Verification items for the finished model (mm, model axes). Face numbers are marked on the shaded views. A direction names the side the tool comes from. Coordinates: 2 decimals unless noted, no trailing zeros. Loops run counter-clockwise (first coordinate to the right, second up) from the corner with the lowest first, then second, coordinate; pieces in that order, holes last.
Q1. Sectioned sample at B-B (x = 10). Enter the section's corners in (y, z).
Q2. Mould release check, pull along X, two halves, no side actions. Record for the marked faces 1, 2 and 3: +X half, -X half, draft (parallel to the pull), parting line (faces both ways), or undercut.
Q3. Sectioned sample at A-A (y = 7.25). Enter the section's corners in (x, z), then the cut area to 3 significant figures.
Q4. Sectioned sample at D-D (x = 20). Enter the section's corners in (y, z), then the cut area to 3 significant figures.
Q5. Material ranges on probe 1 along X at (y, z) = (1, 0); probe 2 along X at (y, z) = (11, 3.55); probe 3 along Z at (x, y) = (6.75, 11.25), recorded low to high.
Q6. Sectioned sample at C-C (y = 3.5). Enter the section's corners in (x, z), then the cut area to 3 significant figures.
Q7. Go/stop test with flat-tipped pins: P1, Ø4, axis at x = 10, y = 11, coming from the +Z side; P2, Ø7, axis at x = 10, y = 11, coming from the -Z side; P3, Ø5, axis at x = 10.5, y = 11, coming from the +Z side; P4, Ø1.5, axis at y = 8, z = 3.5, coming from the +X side. Record where each tip stops, or that it passes through.
Q8. Access from +Z, -Z, +X, -X, +Y, -Y to the whole of each face (thin tool, end or side, straight path). Record for the marked faces 4, 5, 6, 7 and 8.
```python
from build123d import *

# Parameters (mm, degrees)
SKETCH1_W           = 10
SKETCH1_H           = 10
SKETCH1_R           = 2.05
BOSS_EXTRUDE1_DEPTH = 6
CUT_EXTRUDE1_DEPTH  = 3.2
SKETCH3_W           = 10
SKETCH3_H           = 6
BOSS_EXTRUDE2_DEPTH = 20
SKETCH4_R           = 2.05
CUT_EXTRUDE2_DEPTH  = 27.191601707
CUT_EXTRUDE3_DEPTH  = 3.2
SKETCH8_R           = 2.2
BOSS_EXTRUDE4_DEPTH = 4.5
SKETCH10_W          = 17.254554438
SKETCH10_H          = 12.252832867
CUT_EXTRUDE5_DEPTH  = 1.6


with BuildPart() as part:
    # Sketch1 → Boss-Extrude1 (new body)
    with BuildSketch(Plane(origin=(0, 0, 0), x_dir=(1, 0, 0), z_dir=(0, 1, 0))):
        Rectangle(SKETCH1_W, SKETCH1_H)
        with Locations(Location((0, 0, 0), (0, 0, 270))):
            Circle(SKETCH1_R, mode=Mode.SUBTRACT)
    extrude(amount=BOSS_EXTRUDE1_DEPTH)

    # Sketch2 → Cut-Extrude1 (cut)
    with BuildSketch(Plane(origin=(0, 6, 0), x_dir=(1, 0, 0), z_dir=(0, 1, 0))):
        Polygon((4.041451884, 0), (2.020725942, 3.5), (-2.020725942, 3.5), (-4.041451884, 0), (-2.020725942, -3.5), (2.020725942, -3.5), align=None)
    extrude(amount=-CUT_EXTRUDE1_DEPTH, mode=Mode.SUBTRACT)

    # Sketch3 → Boss-Extrude2 (add)
    with BuildSketch(Plane(origin=(5, 0, 0), x_dir=(0, 0, -1), z_dir=(1, 0, 0))):
        with Locations((0, 3)):
            Rectangle(SKETCH3_W, SKETCH3_H)
    extrude(amount=BOSS_EXTRUDE2_DEPTH)

    # Sketch4 → Cut-Extrude2 (cut, through all)
    with BuildSketch(Plane(origin=(0, 6, 0), x_dir=(1, 0, 0), z_dir=(0, 1, 0))):
        with Locations(Location((20, 0, 0), (0, 0, 270))):
            Circle(SKETCH4_R)
    extrude(amount=-CUT_EXTRUDE2_DEPTH, mode=Mode.SUBTRACT)

    # Sketch5 → Cut-Extrude3 (cut)
    with BuildSketch(Plane(origin=(0, 6, 0), x_dir=(1, 0, 0), z_dir=(0, 1, 0))):
        Polygon((24.041451884, 0), (22.020725942, 3.5), (17.979274058, 3.5), (15.958548116, 0), (17.979274058, -3.5), (22.020725942, -3.5), align=None)
    extrude(amount=-CUT_EXTRUDE3_DEPTH, mode=Mode.SUBTRACT)

    # Sketch8 → Boss-Extrude4 (add, symmetric)
    with BuildSketch(Plane.XY):
        with BuildLine():
            Line((5, 6), (5, 11))
            ThreePointArc((5, 11), (10, 16), (15, 11))
            Line((15, 11), (15, 6))
            Line((15, 6), (5, 6))
        make_face()
        with Locations((10, 11)):
            Circle(SKETCH8_R, mode=Mode.SUBTRACT)
    extrude(amount=BOSS_EXTRUDE4_DEPTH, both=True)

    # Sketch10 → Cut-Extrude5 (cut, symmetric)
    with BuildSketch(Plane.XY):
        with Locations((11.441920225, 12.126416434)):
            Rectangle(SKETCH10_W, SKETCH10_H)
    extrude(amount=CUT_EXTRUDE5_DEPTH, both=True, mode=Mode.SUBTRACT)


solid = part.part
```
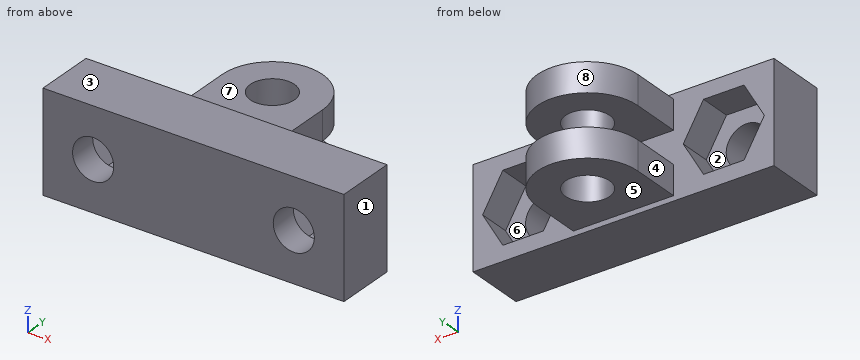
Geometry check:
1. outline: (0, -5) - (6, -5) - (6, -4.5) - (8.8, -4.5) - (8.8, -1.6) - (6, -1.6) - (6, 1.6) - (8.8, 1.6) - (8.8, 4.5) - (6, 4.5) - (6, 5) - (0, 5) - close; (13.2, -4.5) - (16, -4.5) - (16, -1.6) - (13.2, -1.6) - close; (13.2, 1.6) - (16, 1.6) - (16, 4.5) - (13.2, 4.5) - close
2. face 1: +X half
2. face 2: undercut
2. face 3: draft
3. outline: (5, -4.5) - (15, -4.5) - (15, -1.6) - (5, -1.6) - close; (5, 1.6) - (15, 1.6) - (15, 4.5) - (5, 4.5) - close
3. area: 58.0 mm2
4. outline: (0, -5) - (6, -5) - (6, -3.5) - (2.8, -3.5) - (2.8, -2.05) - (0, -2.05) - close; (0, 2.05) - (2.8, 2.05) - (2.8, 3.5) - (6, 3.5) - (6, 5) - (0, 5) - close
4. area: 26.1 mm2
5. probe 1: x = -5 to -2.05, 2.05 to 17.95, 22.05 to 25
5. probe 2: x = 5 to 7.8, 12.2 to 15
5. probe 3: z = -4.5 to -1.6, 1.6 to 4.5
6. outline: (-5, -5) - (25, -5) - (25, 5) - (-5, 5) - close; hole (-4.04, 0) - (-2.02, -3.5) - (2.02, -3.5) - (4.04, 0) - (2.02, 3.5) - (-2.02, 3.5) - close; hole (15.96, 0) - (17.98, -3.5) - (22.02, -3.5) - (24.04, 0) - (22.02, 3.5) - (17.98, 3.5) - close
6. area: 215 mm2
7. P1: passes through
7. P2: stops at z = -4.5
7. P3: stops at z = 4.5
7. P4: stops at x = 15
8. face 4: +Z, -Z, -X, +Y
8. face 5: -Z, +X, -X, +Y
8. face 6: +Y
8. face 7: +Z, +X, -X, +Y
8. face 8: +Z, -Z, +Y
